Input: part model. Units: mm. Frame: model coordinates. A direction names the side the tool comes from. Round coordinates to 2 decimals unless told otherwise and drop trailing zeros.
(1) Draft query along X for faces 4 (the face through (222, 517.5, 0)), 5 (the face through (-20, 542, 0)), 6 (the face through (226, 0, 0)), 7 (the face through (20, 500, 0)). Return one class per face: released by +X, released by -X, zero draft, split by the parting line, or undercut.
(2) Line query: line 1 (X direction, y = 537, z = -1); line 2 (Y direction, x = 386.5, z = -11); line 3 (Y direction, x = 136.5, z = -2). Output: solid intervals per line, ascending.
(3) Access query for faces 1 (the face through (17.5, 523, 0)), 2 (the face through (228, 1030, 0)), 3 (the face through (11, 614, 17.5)). Directions: +Z, -Z, +X, -X, +Y, -Y. A direction counts if a zero-diameter tool reaches every point of the face in a straight line with its end or side. Return the directions, or none.
(4) First-contact query: pin 1 Ø4 at (x, z) = (310, 11.5) entering from -Y; pin 2 Ø1.5 at (y, z) = (501.5, -17) entering from -X; pin 3 Ø4 at (y, z) = (504.5, 17.5) entering from -X. Flat tips, straight axial feed; report the tip coordinate or a pass-through.
(5) Cut plane A-A, the plane y = 193.5. Give the number of separate pieces and of enclosed holes in the cut face, and give its area (3 significant figures).
from build123d import *

# Parameters (mm, degrees)
F5_W     = 150
F5_H     = 6
F6_DEPTH = 410


with BuildPart() as f2:
    # F2: sweep along a path in F1
    with BuildLine(Plane.XY) as f2_path:
        Line((0, 0), (0, 1050))
        Line((0, 1050), (450, 1050))
        Line((450, 1050), (450, 0))
    # F0 (on Front) → F2 (sweep)
    with BuildSketch(Plane.XZ):
        with BuildLine():
            Line((-15, -20), (15, -20))
            ThreePointArc((15, -20), (18.5355339059, -18.5355339059), (20, -15))
            Line((20, -15), (20, 15))
            ThreePointArc((20, 15), (18.5355339059, 18.5355339059), (15, 20))
            Line((15, 20), (-15, 20))
            ThreePointArc((-15, 20), (-18.5355339059, 18.5355339059), (-20, 15))
            Line((-20, 15), (-20, -15))
            ThreePointArc((-20, -15), (-18.5355339059, -18.5355339059), (-15, -20))
        make_face()
        with BuildLine():
            ThreePointArc((-15, -17.5), (-16.767766953, -16.767766953), (-17.5, -15))
            Line((-17.5, -15), (-17.5, 15))
            ThreePointArc((-17.5, 15), (-16.767766953, 16.767766953), (-15, 17.5))
            Line((-15, 17.5), (15, 17.5))
            ThreePointArc((15, 17.5), (16.767766953, 16.767766953), (17.5, 15))
            Line((17.5, 15), (17.5, -15))
            ThreePointArc((17.5, -15), (16.767766953, -16.767766953), (15, -17.5))
            Line((15, -17.5), (-15, -17.5))
        make_face(mode=Mode.SUBTRACT)
    sweep(path=f2_path.line, transition=Transition.RIGHT)

    # F3 (on face) → F4 (join, up to the next surface of F2)
    with BuildSketch(Plane.YZ.offset(20)):
        with BuildLine():
            Line((485, -20), (515, -20))
            ThreePointArc((515, -20), (518.5355339059, -18.5355339059), (520, -15))
            Line((520, -15), (520, 15))
            ThreePointArc((520, 15), (518.5355339059, 18.5355339059), (515, 20))
            Line((515, 20), (485, 20))
            ThreePointArc((485, 20), (481.4644660941, 18.5355339059), (480, 15))
            Line((480, 15), (480, -15))
            ThreePointArc((480, -15), (481.4644660941, -18.5355339059), (485, -20))
        make_face()
        with BuildLine():
            ThreePointArc((485, -17.5), (483.232233047, -16.767766953), (482.5, -15))
            Line((482.5, -15), (482.5, 15))
            ThreePointArc((482.5, 15), (483.232233047, 16.767766953), (485, 17.5))
            Line((485, 17.5), (515, 17.5))
            ThreePointArc((515, 17.5), (516.767766953, 16.767766953), (517.5, 15))
            Line((517.5, 15), (517.5, -15))
            ThreePointArc((517.5, -15), (516.767766953, -16.767766953), (515, -17.5))
            Line((515, -17.5), (485, -17.5))
        make_face(mode=Mode.SUBTRACT)
    extrude(until=Until.NEXT)

    # F5 (on face) → F6 (join, through all)
    with BuildSketch(Plane.YZ.offset(20)):
        with Locations((75, 0)):
            Rectangle(F5_W, F5_H)
    extrude(amount=F6_DEPTH)


solid = f2.part
Reported:
1. face 4: undercut
1. face 5: released by -X
1. face 6: zero draft
1. face 7: undercut
2. line 1: x = -20 to -17.5, 17.5 to 20, 430 to 432.5, 467.5 to 470
2. line 2: y = 480 to 482.5, 517.5 to 520, 1030 to 1032.5, 1067.5 to 1070
2. line 3: y = 0 to 150, 480 to 482.5, 517.5 to 520, 1030 to 1032.5, 1067.5 to 1070
3. face 1: -Y
3. face 2: +Z, -Z
3. face 3: none
4. pin 1: stops at y = 480
4. pin 2: stops at x = -19.84
4. pin 3: stops at x = -19.97
5. separate pieces: 2
5. enclosed holes: 2
5. area: 718 mm2
